Read the model definition and answer for the solid it produces. Units are mm, in the model's axes. Face numbers are marked on the shaded views. A direction names the side the tool comes from. Coordinates: 2 decimals unless noted, no trailing zeros. Write each loop counter-clockwise with the first axis right and the second up, starting at its lowest first coordinate (ties: lowest second). Pieces come first, ordered by that corner, then holes. Notation, with made-up numbers: (84.5, 74.25) -> (100.5, 74.25) arc R18 cw to (100.5, 97.25) -> close; hole circle Ø7 at (-1, 9). An arc over 180 degrees is marked (long way). Answer as a JSON object with one key per item and string values. Group by question number.
(1) Straight lines are drawn through the part: L1, parallel to Z at x = -6.75, y = 6.75; L2, parallel to Y at x = -3.5, z = -10.5; L3, parallel to Y at x = -8.89, z = -1.5. For each, find the intervals that lie inside material, in ascending order.
(2) Which of the six approach directions +Z, -Z, +X, -X, +Y, -Y give full straight-line access (tool end or side, diameter ignored) to the marked faces 1 and 2?
(3) Flat-ended cylindrical pins translate along their axes: P1, Ø4.5, axis at x = 0, z = -30.48, coming from the +Y side; P2, Ø12, axis at x = 6, y = 0.5, coming from the -Z side; P3, Ø2.5, axis at x = 0, y = -8.89, coming from the +Z side. Find the tip coordinate at first contact, or state that the pin passes through.
(4) Find section B-B (x = -8.89). Give the vertices of the cut face in (y, z), then the cut area to 3 significant figures.
(5) Find section A-A (y = -8.89). Give the vertices of the cut face in (x, z), then the cut area to 3 significant figures.
(6) Find section C-C (z = -5.08). Give the vertices of the cut face in (x, y).
(7) Find section D-D (y = -6). Give the vertices of the cut face in (x, z).
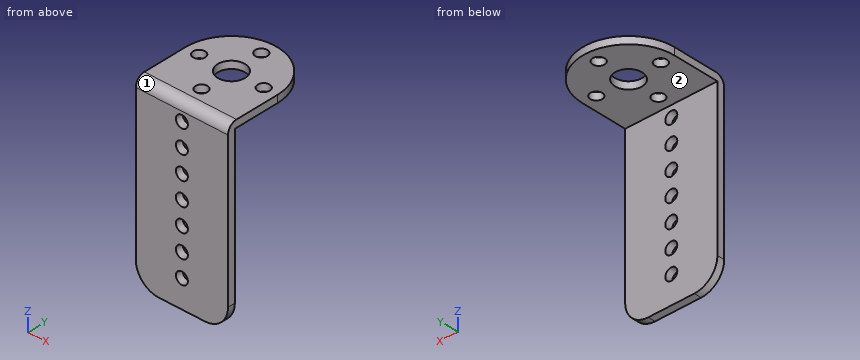
from build123d import *

# Parameters (mm, degrees)
SKETCH1_R           = 3.7465
SKETCH1_R_2         = 1.651
BOSS_EXTRUDE1_DEPTH = 2.032
SKETCH2_W           = 25.4
SKETCH2_H           = 50.8
SKETCH2_R           = 1.651
BOSS_EXTRUDE3_DEPTH = 2.032
FILLET3_R           = 2.54
FILLET4_R           = 6.35


with BuildPart() as part:
    # Sketch1 → Boss-Extrude1 (new body)
    with BuildSketch(Plane.XY):
        with BuildLine():
            Line((-12.7, 0), (-12.7, -14.732))
            Line((-12.7, -14.732), (12.7, -14.732))
            Line((12.7, -14.732), (12.7, 0))
            ThreePointArc((12.7, 0), (0, 12.7), (-12.7, 0))
        make_face()
        Circle(SKETCH1_R, mode=Mode.SUBTRACT)
        with Locations((0, 8.89)):
            Circle(SKETCH1_R_2, mode=Mode.SUBTRACT)
        with Locations((8.89, 0)):
            Circle(SKETCH1_R_2, mode=Mode.SUBTRACT)
        with Locations((0, -8.89)):
            Circle(SKETCH1_R_2, mode=Mode.SUBTRACT)
        with Locations((-8.89, 0)):
            Circle(SKETCH1_R_2, mode=Mode.SUBTRACT)
    extrude(amount=-BOSS_EXTRUDE1_DEPTH)

    # Sketch2 → Boss-Extrude3 (add)
    with BuildSketch(Plane.XZ.offset(14.732)):
        with Locations((0, -25.4)):
            Rectangle(SKETCH2_W, SKETCH2_H)
        with Locations((0, -43.18)):
            Circle(SKETCH2_R, mode=Mode.SUBTRACT)
        with Locations((0, -36.83)):
            Circle(SKETCH2_R, mode=Mode.SUBTRACT)
        with Locations((0, -30.48)):
            Circle(SKETCH2_R, mode=Mode.SUBTRACT)
        with Locations((0, -24.13)):
            Circle(SKETCH2_R, mode=Mode.SUBTRACT)
        with Locations((0, -17.78)):
            Circle(SKETCH2_R, mode=Mode.SUBTRACT)
        with Locations((0, -11.43)):
            Circle(SKETCH2_R, mode=Mode.SUBTRACT)
        with Locations((0, -5.08)):
            Circle(SKETCH2_R, mode=Mode.SUBTRACT)
    extrude(amount=-BOSS_EXTRUDE3_DEPTH)

    # Fillet3
    fillet3_edges = [part.edges().sort_by_distance(p)[0] for p in [
        (0, -14.732, 0),
    ]]
    fillet(fillet3_edges, radius=FILLET3_R)

    # Fillet4
    fillet4_edges = [part.edges().sort_by_distance(p)[0] for p in [
        (-12.7, -13.716, -50.8),
        (12.7, -13.716, -50.8),
    ]]
    fillet(fillet4_edges, radius=FILLET4_R)


solid = part.part
Results below:
{
 "1": {"L1": "z = -2.03 to 0", "L2": "y = -14.73 to -12.7", "L3": "y = -14.51 to -1.65, 1.65 to 9.07"},
 "2": {"face 1": "+Z, +X, -X, -Y", "face 2": "-Z, +X, -X, +Y"},
 "3": {"P1": "stops at y = -12.7", "P2": "stops at z = -2.03", "P3": "passes through"},
 "4": {"outline": "(-14.73, -50.27) -> (-12.7, -50.27) -> (-12.7, -2.03) -> (-1.65, -2.03) -> (-1.65, 0) -> (-12.19, 0) arc R2.54 ccw to (-14.73, -2.54) -> close; (1.65, -2.03) -> (9.07, -2.03) -> (9.07, 0) -> (1.65, 0) -> close", "area": "138 mm2"},
 "5": {"outline": "(-12.7, -2.03) -> (-1.65, -2.03) -> (-1.65, 0) -> (-12.7, 0) -> close; (1.65, -2.03) -> (12.7, -2.03) -> (12.7, 0) -> (1.65, 0) -> close", "area": "44.9 mm2"},
 "6": {"outline": "(-12.7, -14.73) -> (-1.65, -14.73) -> (-1.65, -12.7) -> (-12.7, -12.7) -> close; (1.65, -14.73) -> (12.7, -14.73) -> (12.7, -12.7) -> (1.65, -12.7) -> close"},
 "7": {"outline": "(-12.7, -2.03) -> (12.7, -2.03) -> (12.7, 0) -> (-12.7, 0) -> close"}
}
